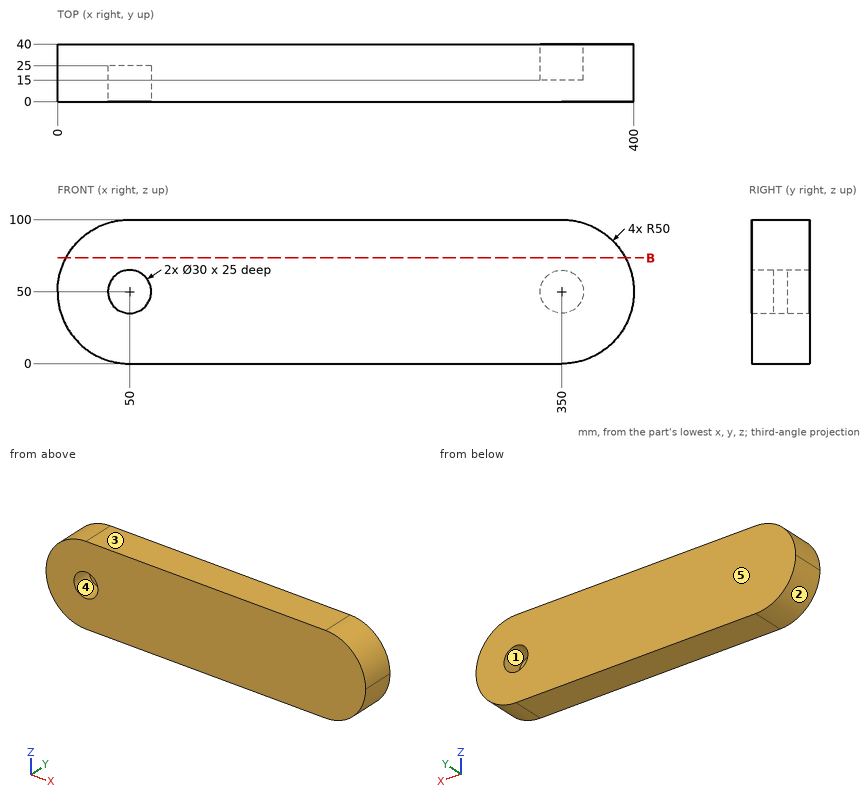
Can you work these out from the drawing? Everything is in mm from the part's minimum corner. A direction names the side the tool comes from. Coordinates: 2 decimals unless noted, no trailing zeros. Order: outer loops, then holes, each group sorted by start corner. A loop starts at its lowest first (then second) coordinate and runs counter-clockwise, first axis right, second up. Notation, with made-up numbers: M -34.5,86 L -25.5,86 A14 ccw -25.5,113 Z; hole C -22.5,39.25 d1. An arc over 180 degrees is marked long. Answer as CSV lines item,"result". Start each with the question number.
1. On a 3-axis mill with a long thin cutter (end or side, diameter ignored), from which of +Z, -Z, +X, -X, +Y, -Y can I reach the whole of each face in a straight line? I mean the marked faces 1 and 2. Say none if no direction works.
2. I want a section at B-B, the plane z = 73.5. Write out the boundary of the cut face in (x, y), and give its area (3 significant figures).
3. We'd pull the mould along Z, two halves only. Please class the marked faces 3, 4 and 5: released by +Z, released by -Z, zero draft, split by the parting line, or undercut.
4. For pin 1 (1 mm diameter, centred on y = 15, z = 84.5, fed in from -X); pin 2 (12 mm diameter, centred on y = 10, z = 66.5, fed in from -X) (3 decimals); pin 3 (1 mm diameter, centred on y = 20, z = 65.5, fed in from -X), each with a flat end and sliding along its axis, tell me the tip position at first contact or that it passes through.
5. I need wall thicknesses on line 1 (X direction, y = 4, z = 50.5); line 2 (X direction, y = 30.5, z = 50); line 3 (Y direction, x = 56.5, z = 59). Which ranges of each line are inside material? Lowest first, please. Write a range as [from, to].
Recorded:
1,face 1,"+Y"
1,face 2,"-Z, -X, +Y, -Y"
2,outline,"M 5.87,0 L 394.13,0 L 394.13,40 L 5.87,40 Z"
2,area,"15,500 mm2"
3,face 3,"released by +Z"
3,face 4,"undercut"
3,face 5,"zero draft"
4,pin 1,"stops at x = 13.34"
4,pin 2,"stops at x = 1.115"
4,pin 3,"stops at x = 2.3"
5,line 1,"x = [0, 35.01], [64.99, 400]"
5,line 2,"x = [0, 335], [365, 400]"
5,line 3,"y = [25, 40]"
